Could you check a few things on this model? Use its own coordinates, in mm. A direction names the side the tool comes from. Give positions to 0.01 mm unless a question says otherwise; leave off trailing zeros. Order: outer loops, then holes, each group sorted by start corner. A loop starts at its lowest first (then second) coordinate and runs counter-clockwise, first axis right, second up. Notation, with made-up numbers: (83.25, 16.5) - (131.25, 16.5) arc R31 ccw to (131.25, 41.5) - close; hole circle Ø11 at (72, 61.25). An arc over 180 degrees is marked (long way). Put each result on its own line as item: value.
from build123d import *

# Parameters (mm, degrees)
PAD018_DEPTH            = 16
PAD019_DEPTH            = 1
SKETCH049_R             = 6
SKETCH049_R_2           = 1.5
POCKET012_DEPTH         = 5
SKETCH050_R             = 2.5
SKETCH050_W             = 6
SKETCH050_H             = 5
POCKET013_DEPTH         = 2
SKETCH051_R             = 2.25
SKETCH051_R_2           = 2.5
PAD020_DEPTH            = 17
SKETCH053_W             = 46
SKETCH053_H             = 22
PAD021_DEPTH            = 6
SKETCH054_R             = 2.25
POCKET015_DEPTH         = 8
POCKET016_DEPTH         = 4
SKETCH065_W             = 14
SKETCH065_H             = 6
POCKET023_DEPTH         = 8
POCKET080_DEPTH         = 4
BODY007_PLACEMENT_ANGLE = 180


with BuildPart() as part:
    # Sketch046 → Pad018 (new body)
    with BuildSketch(Plane.XY):
        with BuildLine():
            Line((-13.5, 0), (-13.5, -72.44))
            ThreePointArc((-13.5, -72.44), (-11.57862, -77.07862), (-6.94, -79))
            Line((-6.94, -79), (6.94, -79))
            ThreePointArc((6.94, -79), (11.57862, -77.07862), (13.5, -72.44))
            Line((13.5, -72.44), (13.5, 0))
            Line((13.5, 0), (-13.5, 0))
        make_face()
        with BuildLine():
            Line((11.5, -2), (11.5, -72))
            ThreePointArc((6.5, -77), (10.035534, -75.535534), (11.5, -72))
            Line((6.5, -77), (-6.5, -77))
            ThreePointArc((-11.5, -72), (-10.035534, -75.535534), (-6.5, -77))
            Line((-11.5, -72), (-11.5, -2))
            Line((-11.5, -2), (11.5, -2))
        make_face(mode=Mode.SUBTRACT)
    extrude(amount=PAD018_DEPTH)

    # Sketch047 (on Face14 of Pad018) → Pad019 (join)
    with BuildSketch(Plane.XY.offset(16)):
        with BuildLine():
            Line((-13.5, 0), (13.5, 0))
            Line((13.5, 0), (13.5, -72.44))
            ThreePointArc((6.94, -79), (11.57862, -77.07862), (13.5, -72.44))
            Line((6.94, -79), (-6.94, -79))
            ThreePointArc((-13.5, -72.44), (-11.57862, -77.07862), (-6.94, -79))
            Line((-13.5, -72.44), (-13.5, 0))
        make_face()
    extrude(amount=PAD019_DEPTH)

    # Sketch049 → Pocket012 (cut)
    with BuildSketch(Plane.XY.offset(17)):
        with Locations((0, -65.5)):
            Circle(SKETCH049_R)
        with Locations((8, -45)):
            Circle(SKETCH049_R_2)
        with Locations((-8, -45)):
            Circle(SKETCH049_R_2)
    extrude(amount=-POCKET012_DEPTH, mode=Mode.SUBTRACT)

    # Sketch050 (on Face21 of Pocket012) → Pocket013 (cut)
    with BuildSketch(Plane(origin=(0, 0, 16), x_dir=(1, 0, 0), z_dir=(0, 0, -1))):
        with Locations((0, 54)):
            Circle(SKETCH050_R)
        with Locations((0, 33.5)):
            Rectangle(SKETCH050_W, SKETCH050_H)
    extrude(amount=-POCKET013_DEPTH, mode=Mode.SUBTRACT)

    # Sketch051 (on Face17 of Pocket013) → Pad020 (join)
    with BuildSketch(Plane.XY.offset(17)):
        with BuildLine():
            Line((-13, -49), (-13, -59))
            Line((-13, -59), (-18, -59))
            ThreePointArc((-18, -49), (-23.000001, -54), (-18, -59))
            Line((-13, -49), (-18, -49))
        make_face()
        with Locations((-18.000001, -54)):
            Circle(SKETCH051_R, mode=Mode.SUBTRACT)
        with BuildLine():
            Line((13, -49), (13, -59))
            Line((13, -59), (18, -59))
            ThreePointArc((18, -59), (23, -54), (18, -49))
            Line((13, -49), (18, -49))
        make_face()
        with Locations((18, -54)):
            Circle(SKETCH051_R, mode=Mode.SUBTRACT)
        with BuildLine():
            Line((13, -10), (13, -20))
            Line((13, -20), (18, -20))
            ThreePointArc((18, -20), (23, -15), (18, -10))
            Line((13, -10), (18, -10))
        make_face()
        with Locations((18, -15)):
            Circle(SKETCH051_R, mode=Mode.SUBTRACT)
        with BuildLine():
            Line((-13, -10), (-13, -20))
            Line((-13, -20), (-18, -20))
            ThreePointArc((-18, -10), (-22.999995, -15), (-18, -20))
            Line((-13, -10), (-18, -10))
        make_face()
        with Locations((-17.999995, -15)):
            Circle(SKETCH051_R_2, mode=Mode.SUBTRACT)
    extrude(amount=-PAD020_DEPTH)

    # Sketch053 (on Face5 of Pad020) → Pad021 (join)
    with BuildSketch(Plane(origin=(0, 0, 0), x_dir=(-1, 0, 0), z_dir=(0, 1, 0))):
        with Locations((0, 6)):
            Rectangle(SKETCH053_W, SKETCH053_H)
    extrude(amount=PAD021_DEPTH)

    # Sketch054 (on Face64 of Pad021) → Pocket015 (cut)
    with BuildSketch(Plane(origin=(0, 6, 0), x_dir=(-1, 0, 0), z_dir=(0, 1, 0))):
        with Locations((-18, 6)):
            Circle(SKETCH054_R)
        with Locations((18, 6)):
            Circle(SKETCH054_R)
    extrude(amount=-POCKET015_DEPTH, mode=Mode.SUBTRACT)

    # Sketch055 (on Face5 of Pocket015) → Pocket016 (cut)
    with BuildSketch(Plane.XZ):
        Polygon((-14.535898, 4), (-14.535898, 8), (-18, 10), (-21.464102, 8), (-21.464102, 4), (-18, 2), align=None)
        Polygon((21.464102, 4), (21.464102, 8), (18, 10), (14.535898, 8), (14.535898, 4), (18, 2), align=None)
    extrude(amount=-POCKET016_DEPTH, mode=Mode.SUBTRACT)

    # Sketch065 (on Face76 of Pocket016) → Pocket023 (cut)
    with BuildSketch(Plane(origin=(0, 6, 0), x_dir=(-1, 0, 0), z_dir=(0, 1, 0))):
        with Locations((0, 6)):
            Rectangle(SKETCH065_W, SKETCH065_H)
    extrude(amount=-POCKET023_DEPTH, mode=Mode.SUBTRACT)

    # Sketch056 (on Face86 of Pocket023) → Pocket080 (cut)
    with BuildSketch(Plane.XY.offset(17)):
        Polygon((-14.535898, -56), (-14.535898, -52), (-18, -50), (-21.464102, -52), (-21.464102, -56), (-18, -58), align=None)
        Polygon((21.464102, -56), (21.464102, -52), (18, -50), (14.535898, -52), (14.535898, -56), (18, -58), align=None)
        Polygon((21.464102, -17), (21.464102, -13), (18, -11), (14.535898, -13), (14.535898, -17), (18, -19), align=None)
        Polygon((-14.535898, -17), (-14.535898, -13), (-18, -11), (-21.464102, -13), (-21.464102, -17), (-18, -19), align=None)
    extrude(amount=-POCKET080_DEPTH, mode=Mode.SUBTRACT)


with BuildPart() as part_1:
    # Body007 placement: moved
    add(part.part.moved(Location((0, -40, 3))).rotate(Axis((0, -40, 3), (0, 1, 0)), BODY007_PLACEMENT_ANGLE))


solid = part_1.part
1) Which directions (+Z, -Z, +X, -X, +Y, -Y) give clear straight access to the entire face, cutting with the end or side of a thin tool? Please do faces 1 (the flat face through (13.5, -45, -5)), 2 (the flat face through (16.244, -52.014, -12.028)), 3 (the flat face through (-19.756, -38.028, -5.986)), 4 (the flat face through (13.5, -106, -5)).
Filled in:
face 1: +Z, -Z, +X
face 2: -Z
face 3: none
face 4: +Z, -Z, +X, -Y
2) I'm going to push flat-ended pins straight in: pin 1 (12 mm diameter, centred on y = -87, z = -5, fed in from -X); pin 2 (0.5 mm diameter, centred on y = -74, z = -13.5, fed in from -X); pin 3 (8 mm diameter, centred on y = -88, z = -3, fed in from +X). Where does each tip first touch, or does it pass through?
Filled in:
pin 1: stops at x = -22.9
pin 2: stops at x = -13.5
pin 3: stops at x = 22.58
3) If I drill on line 1 (Y direction, x = -21, z = -3); line 2 (X direction, y = -94, z = -2.5); line 3 (X direction, y = -85, z = -13.75), over which ranges is the centre line in solid material (lowest first)? Write a range as [from, to].
Filled in:
line 1: y = [-98, -90], [-59, -51], [-36, -34]
line 2: x = [-23, -20.25], [-15.75, -11.5], [11.5, 15.75], [20.25, 23]
line 3: x = [-13.5, -9.5], [-6.5, 6.5], [9.5, 13.5]
4) We'd pull the mould along Z, two halves only. Please class faces 5 (the flat face through (-13.5, -106, -5)), 6 (the flat face through (7, -38, -3)), 7 (the flat face through (0, -37, 8)): pulls with the +Z half, pulls with the -Z half, needs draft (parallel to the pull), parting line crosses it, or undercut.
Filled in:
face 5: needs draft
face 6: undercut
face 7: pulls with the +Z half
5) Suppose I cut it at A-A, the plane y = -105.5. List the corners of the cut face in (x, z) for me.
Filled in:
outline: (-13.5, -14) - (-6, -14) - (-6, -13) - (-11.5, -13) - (-11.5, 3) - (-13.5, 3) - close; (6, -14) - (13.5, -14) - (13.5, 3) - (11.5, 3) - (11.5, -13) - (6, -13) - close
6) Suppose I cut it at C-C, the plane y = -85. List the corners of the cut face in (x, z) for me.
Filled in:
outline: (-13.5, -14) - (-9.5, -14) - (-9.5, -13) - (-11.5, -13) - (-11.5, 3) - (-13.5, 3) - close; (-6.5, -14) - (6.5, -14) - (6.5, -13) - (-6.5, -13) - close; (9.5, -14) - (13.5, -14) - (13.5, 3) - (11.5, 3) - (11.5, -13) - (9.5, -13) - close
7) Suppose I cut it at B-B, the plane x = 0. List the corners of the cut face in (y, z) for me.
Filled in:
outline: (-119, -14) - (-111.5, -14) - (-111.5, -13) - (-117, -13) - (-117, 3) - (-119, 3) - close; (-99.5, -14) - (-96.5, -14) - (-96.5, -13) - (-99.5, -13) - close; (-91.5, -14) - (-76, -14) - (-76, -13) - (-91.5, -13) - close; (-71, -14) - (-34, -14) - (-34, -6) - (-42, -6) - (-42, -13) - (-71, -13) - close; (-42, 0) - (-34, 0) - (-34, 8) - (-40, 8) - (-40, 3) - (-42, 3) - close
8) Suppose I cut it at D-D, the plane z = -3. State how many separate pieces and enclosed holes the cut face has, and give its area (3 significant figures).
Filled in:
separate pieces: 3
enclosed holes: 4
area: 761 mm^2
